Autodesk Inventor part; units mm, degrees
ref_plane "YZ Plane" through (0, 0, 0) normal (1, 0, 0) x (0, 1, 0)
ref_plane "XZ Plane" through (0, 0, 0) normal (0, 1, 0) x (-1, 0, 0)
ref_plane "XY Plane" through (0, 0, 0) normal (0, 0, 1) x (1, 0, 0)
sketch "Sketch1" plane through (0, 0, 0) normal (0, 0, 1) x (1, 0, 0)
  line L0 (-30, 30) -> (30, 30)
  line L1 (30, 30) -> (30, -30)
  line L2 (30, -30) -> (-30, -30)
  line L3 (-30, -30) -> (-30, 30)
  point P0 (0, 0)
  dimension "d0" = 60
  dimension "d1" = 60
  dimension "d2" = 30
  dimension "d3" = 30
extrude "Extrusion1" add sketch "Sketch1" along normal blind 5
sketch "Sketch2" plane through (0, 0, 5) normal (0, 0, 1) x (1, 0, 0)
  line L0 (-26.5, 26.5) -> (26.5, 26.5)
  line L1 (26.5, 26.5) -> (26.5, -26.5)
  line L2 (26.5, -26.5) -> (-26.5, -26.5)
  line L3 (-26.5, -26.5) -> (-26.5, 26.5)
  line L4 (30, 30) -> (-30, 30)
  line L5 (30, -30) -> (30, 30)
  line L6 (-30, 30) -> (30, 30)
  line L7 (30, 30) -> (30, -30)
  line L8 (30, -30) -> (-30, -30)
  line L9 (-30, -30) -> (-30, 30)
  point P0 (0, 0)
  dimension "d6" = 53
  dimension "d7" = 53
  dimension "d8" = 26.5
  dimension "d9" = 26.5
extrude "Extrusion2" add sketch "Sketch2" along normal blind 40
sketch "Sketch3" plane through (-30, -30, 0) normal (0, -1, 0) x (1, 0, 0)
  circle A0 centre (30, 23.5) radius 18.5
  point P0 (30, 0)
  dimension "d12" = 37
  dimension "d13" = 23.5
extrude "Extrusion3" cut sketch "Sketch3" against normal blind 2
sketch "Sketch4" plane through (0, -28, 23.5) normal (0, -1, 0) x (1, 0, 0)
  circle A0 centre (0, 0) radius 9.75
  circle A1 centre (0, 0) radius 18.5
  point P0 (0, -23.5)
  dimension "d19" = 19.5
extrude "Extrusion4" cut sketch "Sketch4" against normal blind 2 contours A0
pattern_circular "Circular Pattern2" count 4 over 360 about axis through (0, 0, -10) along (0, 0, 1) of "Extrusion4"
mirror "Mirror1" about plane through (0, 0, 0) normal (0, 1, 0) of "Extrusion3"
sketch "Sketch6" plane through (30, -30, 0) normal (1, 0, 0) x (0, 0, -1)
  circle A0 centre (-23.5, 30) radius 12.5
  circle A1 centre (-23.5, 30) radius 9.75
  point P0 (0, 30)
  dimension "d28" = 25
extrude "Extrusion6" cut sketch "Sketch6" against normal blind 2 contours A0 | A1
mirror "Mirror2" about plane through (0, 0, 0) normal (1, 0, 0) of "Extrusion6"
properties part number "sampleChamber_singlePiece_filipeSample_V1"
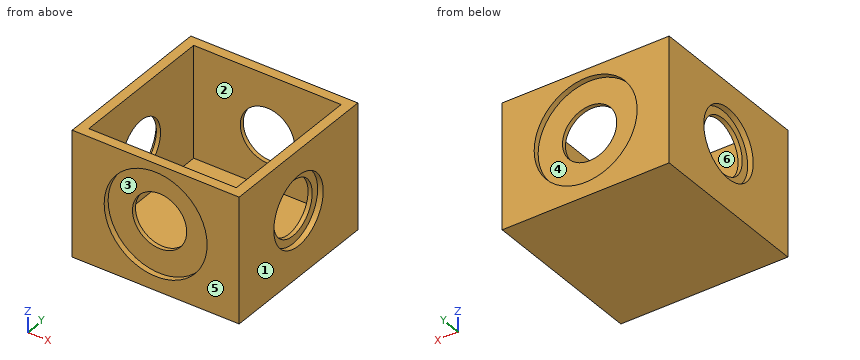
CAD build for the part. Positions are in the model's coordinates, mm. Face numbers are marked on the shaded views. A direction names the side the tool comes from. Round coordinates to 2 decimals unless told otherwise and drop trailing zeros. Write each loop counter-clockwise with the first axis right and the second up, starting at its lowest first coordinate (ties: lowest second). Pieces come first, ordered by that corner, then holes.
Item 1: Band-saw the part on C-C on z = 23.5. Give the number of separate pieces and of enclosed holes in the cut face, then the cut area to 3 significant figures.
Filled in:
separate pieces: 4
enclosed holes: 0
area: 426 mm2
Item 2: Band-saw the part on D-D on x = -25. Write the cut outline in (y, z).
Filled in:
outline: (-30, 0) - (30, 0) - (30, 45) - (26.5, 45) - (26.5, 5) - (-26.5, 5) - (-26.5, 45) - (-30, 45) - close
Item 3: Tool access for the marked faces 1, 2 and 3: list every direction of +Z, -Z, +X, -X, +Y, -Y with a clear straight run to the whole face (end or side of a thin tool).
Filled in:
face 1: +Z, -Z, +X, +Y, -Y
face 2: +Z
face 3: -Y
Item 4: Band-saw the part on B-B on x = 0. Write the cut outline in (y, z).
Filled in:
outline: (-30, 0) - (30, 0) - (30, 5) - (28, 5) - (28, 13.75) - (26.5, 13.75) - (26.5, 5) - (-26.5, 5) - (-26.5, 13.75) - (-28, 13.75) - (-28, 5) - (-30, 5) - close; (-30, 42) - (-28, 42) - (-28, 33.25) - (-26.5, 33.25) - (-26.5, 45) - (-30, 45) - close; (26.5, 33.25) - (28, 33.25) - (28, 42) - (30, 42) - (30, 45) - (26.5, 45) - close
Item 5: Mould opens along Y. For the marked faces 4, 5 and 6 say: released by +Y, released by -Y, zero draft, split by the parting line, or undercut.
Filled in:
face 4: released by +Y
face 5: released by -Y
face 6: undercut
Item 6: Band-saw the part on A-A on y = 0. Write the cut outline in (x, z), then the cut area to 4 significant figures.
Filled in:
outline: (-30, 0) - (30, 0) - (30, 11) - (28, 11) - (28, 13.75) - (26.5, 13.75) - (26.5, 5) - (-26.5, 5) - (-26.5, 13.75) - (-28, 13.75) - (-28, 11) - (-30, 11) - close; (-30, 36) - (-28, 36) - (-28, 33.25) - (-26.5, 33.25) - (-26.5, 45) - (-30, 45) - close; (26.5, 33.25) - (28, 33.25) - (28, 36) - (30, 36) - (30, 45) - (26.5, 45) - close
area: 421.5 mm2
Item 7: Drill centre lines: L1, parallel to X at y = 26, z = 23; L2, parallel to Z at x = 0, y = -27.7; L3, parallel to Y at x = 2, z = 7. Where is each one in solid material? Low to high.
Filled in:
L1: x = -30 to -26.5, 26.5 to 30
L2: z = 0 to 13.75, 33.25 to 45
L3: y = -28 to -26.5, 26.5 to 28
Item 8: Drop flat-ended pins along their axis: pin 1 Ø15 at (y, z) = (0, 23.5) entering from -X; pin 2 Ø22.5 at (y, z) = (0, 23.5) entering from -X; pin 3 Ø11 at (x, z) = (1.5, 17) entering from +Y; pin 4 Ø1 at (x, z) = (-7.5, 15) entering from -Y. Give the stop position or say it passes through.
Filled in:
pin 1: passes through
pin 2: stops at x = -28
pin 3: stops at y = 28
pin 4: stops at y = -28
